Source: CAD feature listing. Evaluate the final solid. Frame: model axes, mm. A direction names the side the tool comes from. Round coordinates to 2 decimals unless told otherwise and drop trailing zeros. Loops run counter-clockwise (first coordinate to the right, second up) from the corner with the lowest first, then second, coordinate; pieces in that order, holes last. Notation, with made-up numbers: (31, -24) -> (53, -24) arc R16 ccw to (53, -13) -> close; hole circle Ø8 at (69.5, -30.75). An arc over 180 degrees is marked (long way). Put each result on its own line as item: value. Start each with the question number.
1. Draft query along Y for faces 4 (the flat face through (-22, 11, 12)), 5 (the cylindrical face through (-18.28, -30.736, -4.036)), 6 (the flat face through (24, 20.2, 0.4)). Return one class per face: pulls with the +Y half, pulls with the -Y half, needs draft (parallel to the pull), parting line crosses it, or undercut.
2. Cut plane B-B (x = 25). Return the cut outline in (y, z).
3. Contact query for flat-ended pins moving along their axis: pin 1 (2 mm diameter, centred on y = 8, z = -3.5, fed in from -X); pin 2 (10 mm diameter, centred on x = -32, z = 12, fed in from +Y); pin 3 (6 mm diameter, centred on x = -3.5, y = 14.5, fed in from -Z). Output: stop coordinate, or through.
4. Material intervals for L1, parallel to X at y = -3, z = -18.5; L2, parallel to Y at x = -24, z = 0; L3, parallel to Y at x = -34.25, z = 0, sorted ascending.
5. Cut plane A-A (x = -37). Return the cut outline in (y, z), then the cut area to 3 significant figures.
6. Set-up query: faces 1 (the cylindrical face through (-25.451, 7.852, 18.937)), 2 (the cylindrical face through (42.48, 15.62, -3.47)), 3 (the cylindrical face through (-37.18, 15.62, -3.47)). Return all of +Z, -Z, +X, -X, +Y, -Y with unobstructed straight access to the full face (end or side cutting, diameter ignored); none if empty.
```python
from build123d import *

# Parameters (mm, degrees)
FILLET3_R = 6


with BuildPart() as part:
    # Sketch1 → Revolve1 (revolve)
    with BuildSketch(Plane.XY, mode=Mode.PRIVATE) as revolve1_sk:
        with BuildLine():
            Line((44, 6), (44, 16))
            Line((44, 16), (41, 16))
            Line((41, 16), (41, 20))
            Line((41, 20), (24, 20))
            Line((24, 20), (24, 31))
            Line((24, 31), (10, 31))
            ThreePointArc((10, 31), (6, 27), (2, 31))
            Line((2, 31), (-44, 31))
            Line((-44, 31), (-44, 25))
            Line((-44, 25), (-42.5, 25))
            Line((-42.5, 25), (-42.5, 16))
            Line((-42.5, 16), (-32, 16))
            Line((-32, 16), (-32, 12.5))
            Line((-32, 12.5), (-29, 12.5))
            Line((-29, 12.5), (-29, 20.5))
            Line((-29, 20.5), (-22, 20.5))
            Line((-22, 20.5), (-22, 16))
            Line((-22, 16), (-14, 16))
            Line((-14, 16), (-14, 6))
            Line((-14, 6), (44, 6))
        make_face()
    revolve(revolve1_sk.sketch.rotate(Axis((-44, 0, 0), (1, 0, 0)), 90), axis=Axis((-44, 0, 0), (1, 0, 0)))

    # Fillet3
    fillet3_edges = [part.edges().sort_by_distance(p)[0] for p in [
        (-44, 0, -31),
    ]]
    fillet(fillet3_edges, radius=FILLET3_R - 0.0001)  # a hair under: the kernel refuses the full size


solid = part.part
```
Solution:
1. face 4: undercut
1. face 5: parting line crosses it
1. face 6: needs draft
2. outline: circle Ø40 at (0, 0); hole circle Ø12 at (0, 0)
3. pin 1: stops at x = -14
3. pin 2: stops at y = 30.2
3. pin 3: stops at z = -28.79
4. L1: x = -42.5 to -29, -22 to 41
4. L2: y = -31 to -20.5, 20.5 to 31
4. L3: y = -31 to -16, 16 to 31
5. outline: circle Ø62 at (0, 0); hole circle Ø32 at (0, 0)
5. area: 2,210 mm^2
6. face 1: none
6. face 2: +X
6. face 3: -X
